```python
from build123d import *

# Parameters (mm, degrees)
AUFSATZ_LINEAR_AUSTRAGEN1_DEPTH             = 2
FORMSENKUNG_F_R_M4_SENKSCHRAUBE_MIT_2_COUNT = 2
FORMSENKUNG_F_R_M4_SENKSCHRAUBE_MIT_2_PITCH = 470
SKIZZE4_R                                   = 1.7
SKIZZE4_W                                   = 23
SKIZZE4_H                                   = 17
SKIZZE4_W_2                                 = 20
SKIZZE4_H_2                                 = 1
SCHNITT_LINEAR_AUSTRAGEN1_DEPTH             = 10
SKIZZE7_W                                   = 500
SKIZZE7_H                                   = 8
SCHNITT_LINEAR_AUSTRAGEN3_DEPTH             = 10


with BuildPart() as part:
    # Skizze1 → Aufsatz-Linear austragen1 (new body)
    with BuildSketch(Plane.XY):
        Polygon((-339.903846154, 3), (160.096153846, 3), (160.096153846, -63), (130.094653846, -63), (130.094653846, -71), (-309.902346154, -71), (-309.902346154, -63), (-316.903846154, -63), (-339.903846154, -63), align=None)
    extrude(amount=AUFSATZ_LINEAR_AUSTRAGEN1_DEPTH)

    # Skizze3 → Formsenkung für M4 Senkschraube mit Innensechskant1 (revolve, cut)
    with BuildSketch(Plane(origin=(145.096153846, -30, 2), x_dir=(0, -1, 0), z_dir=(1, 0, 0))):
        Polygon((0, 0), (0, 2), (2.25, 2), (2.25, 2.05), (4.3, 0), align=None)
    formsenkung_f_r_m4_senkschraube_mit_inne = revolve(axis=Axis((145.096153846, -30, 8.35), (0, 0, -1)), mode=Mode.SUBTRACT)

    # Formsenkung f_r M4 Senkschraube mit  2: Formsenkung für M4 Senkschraube mit Innensechskant1 ×2
    with Locations(*[(-i * FORMSENKUNG_F_R_M4_SENKSCHRAUBE_MIT_2_PITCH, 0, 0) for i in range(1, FORMSENKUNG_F_R_M4_SENKSCHRAUBE_MIT_2_COUNT)]):
        add(formsenkung_f_r_m4_senkschraube_mit_inne, mode=Mode.SUBTRACT)

    # Skizze4 → Schnitt-Linear austragen1 (cut)
    with BuildSketch(Plane.XY.offset(2)):
        with Locations((-268.903846154, -47.5)):
            Circle(SKIZZE4_R)
        with Locations((-297.903846154, -47.5)):
            Circle(SKIZZE4_R)
        with Locations((-218.903846154, -47.5)):
            Circle(SKIZZE4_R)
        with Locations((-247.903846154, -47.5)):
            Circle(SKIZZE4_R)
        with Locations((-283.403846154, -47.5)):
            Rectangle(SKIZZE4_W, SKIZZE4_H)
        with Locations((-179.903846154, -47)):
            Rectangle(SKIZZE4_W_2, SKIZZE4_H_2)
        with Locations((-233.403846154, -47.5)):
            Rectangle(SKIZZE4_W, SKIZZE4_H)
    extrude(amount=-SCHNITT_LINEAR_AUSTRAGEN1_DEPTH, mode=Mode.SUBTRACT)

    # Skizze7 → Schnitt-Linear austragen3 (cut)
    with BuildSketch(Plane(origin=(0, 0, 0), x_dir=(-1, 0, 0), z_dir=(0, 0, -1))):
        with Locations((89.903846154, -67)):
            Rectangle(SKIZZE7_W, SKIZZE7_H)
    extrude(amount=-SCHNITT_LINEAR_AUSTRAGEN3_DEPTH, mode=Mode.SUBTRACT)


solid = part.part
```
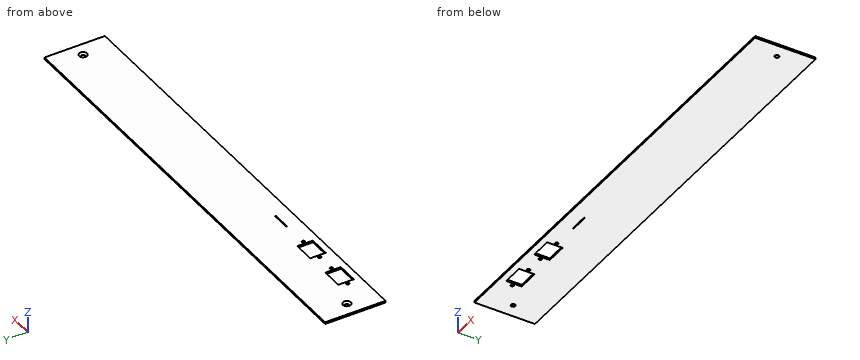
Verification items for the finished model (mm, model axes). Coordinates: 2 decimals unless noted, no trailing zeros. Answer in a Markdown table with one row per item.
1) Section check A-A (z = 1.35). Give the number of separate pieces and of enclosed holes in the cut face, and give its area (3 significant figures).
The answers:
| item | result |
|---|---|
| separate pieces | 1 |
| enclosed holes | 9 |
| area | 32,100 mm2 |
2) Depth check by flat-ended pin: P1, Ø5, axis at x = -159.5, y = -13, coming from the -Z side. Enter the tip coordinate at first touch or a pass-through.
The answers:
| item | result |
|---|---|
| P1 | stops at z = 0 |
3) Scan lines: line 1 along X through (y, z) = (-53.5, 0.2); line 2 along X through (y, z) = (-27, 1.6). Record each from-to range of solid material in increasing order. Write a range as from..to.
The answers:
| item | result |
|---|---|
| line 1 | x = -339.9..-294.9, -271.9..-244.9, -221.9..160.1 |
| line 2 | x = -339.9..-327.4, -322.41..142.6, 147.59..160.1 |
